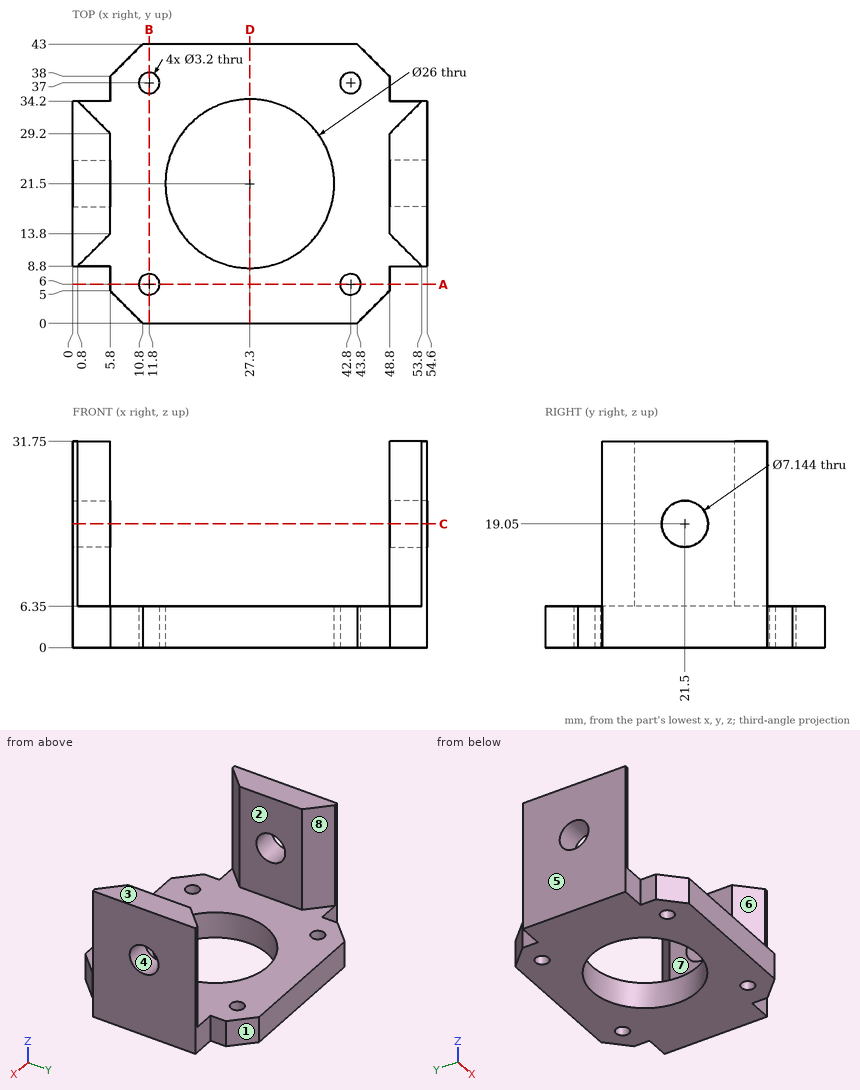
Answer from the drawing. Dimensions are ordinates in mm from the lowest x, y and z of the part. A direction names the side the tool comes from. Round coordinates to 2 decimals unless told otherwise and drop trailing zeros. Loops run counter-clockwise (first coordinate to the right, second up) from the corner with the lowest first, then second, coordinate; pieces in that order, holes last. Notation, with made-up numbers: (25, 15.25) - (66, 15.25) arc R12 ccw to (66, 25.25) - close; hole circle Ø6 at (-21.5, 68). An arc over 180 degrees is marked (long way). Return JSON: item names as keys, results as strings. Group by question number.
1. The part is cut by section D-D on x = 27.3. Determine the outline of the cut face in (y, z), then the cut area to 3 significant figures.
2. Which of the six approach directions +Z, -Z, +X, -X, +Y, -Y give full straight-line access (tool end or side, diameter ignored) to the marked faces 4, 5, 6, 7 and 8?
3. The part is cut by section A-A on y = 6. Determine the outline of the cut face in (x, z).
4. Each of these flat-tipped pins is pushed along its axis until it touches: P1, Ø5, axis at x = 42.8, y = 6, coming from the -Z side; P2, Ø5.5, axis at y = 21.5, z = 19.05, coming from the +X side; P3, Ø3, axis at x = 51.5, z = 16.5, coming from the +Y side; P4, Ø1.1, axis at y = 36, z = 2.5, coming from the +X side. Where does it stop, or does it pass through?
5. The mould has two halves that part along X. Classify the marked faces 1, 2 and 3: pulls with the +X half, pulls with the -X half, needs draft (parallel to the pull), parting line crosses it, or undercut.
6. The part is cut by section C-C on z = 19.05. Determine the outline of the cut face in (x, y).
7. Consider probe 1 along Y at (x, z) = (11.8, 2.5); probe 2 along X at (y, z) = (21, 1); probe 3 along X at (y, z) = (5.5, 5). Determine where each line is inside the solid, lowest interval first.
8. The part is cut by section B-B on x = 11.8. Determine the outline of the cut face in (y, z), then the cut area to 3 significant figures.
Resolved:
{
 "1": {"outline": "(0, 0) - (8.5, 0) - (8.5, 6.35) - (0, 6.35) - close; (34.5, 0) - (43, 0) - (43, 6.35) - (34.5, 6.35) - close", "area": "108 mm²"},
 "2": {"face 4": "+X, -X", "face 5": "+Z, -Z, -X, +Y, -Y", "face 6": "+Z, -Y", "face 7": "+Z, +Y, -Y", "face 8": "+Z, +Y"},
 "3": {"outline": "(5.8, 0) - (10.2, 0) - (10.2, 6.35) - (5.8, 6.35) - close; (13.4, 0) - (41.2, 0) - (41.2, 6.35) - (13.4, 6.35) - close; (44.4, 0) - (48.8, 0) - (48.8, 6.35) - (44.4, 6.35) - close"},
 "4": {"P1": "stops at z = 0", "P2": "passes through", "P3": "stops at y = 33.4", "P4": "stops at x = 48.8"},
 "5": {"face 1": "pulls with the +X half", "face 2": "undercut", "face 3": "needs draft"},
 "6": {"outline": "(0, 8.8) - (0.8, 8.8) - (5.8, 13.8) - (5.8, 17.93) - (0, 17.93) - close; (0, 25.07) - (5.8, 25.07) - (5.8, 29.2) - (0.8, 34.2) - (0, 34.2) - close; (48.8, 13.8) - (53.8, 8.8) - (54.6, 8.8) - (54.6, 17.93) - (48.8, 17.93) - close; (48.8, 25.07) - (54.6, 25.07) - (54.6, 34.2) - (53.8, 34.2) - (48.8, 29.2) - close"},
 "7": {"probe 1": "y = 0 to 4.4, 7.6 to 35.4, 38.6 to 43", "probe 2": "x = 0 to 14.31, 40.29 to 54.6", "probe 3": "x = 5.8 to 10.28, 13.32 to 41.28, 44.32 to 48.8"},
 "8": {"outline": "(0, 0) - (4.4, 0) - (4.4, 6.35) - (0, 6.35) - close; (7.6, 0) - (35.4, 0) - (35.4, 6.35) - (7.6, 6.35) - close; (38.6, 0) - (43, 0) - (43, 6.35) - (38.6, 6.35) - close", "area": "232 mm²"}
}
